Verification items for the finished model (mm, model axes). A direction names the side the tool comes from. Coordinates: 2 decimals unless noted, no trailing zeros. Order: outer loops, then holes, each group sorted by start corner. A loop starts at its lowest first (then second) coordinate and runs counter-clockwise, first axis right, second up. Notation, with made-up numbers: (55, -3) - (68, -3) arc R28 ccw to (68, 36) - close; hole circle Ø1 at (24, 67). An arc over 180 degrees is marked (long way). Answer as CSV lines item,"result". Start each with the question number.
1. Material ranges on L1, parallel to Y at x = 21.05, z = -28.5; L2, parallel to X at y = 9, z = -33; L3, parallel to Z at x = -3.5, y = 6.75, recorded low to high. Write a range as [from, to].
2. Section check C-C (z = -28.5). Record the cut outline in (x, y), and give its area (3 significant figures).
3. Section check A-A (z = -15.5). Record the cut outline in (x, y).
4. Section check B-B (y = 12.5). Record the cut outline in (x, z).
5. Set-up check for faces 4 (the cylindrical face through (20.857, 18.835, -32.206)), 5 (the cylindrical face through (-20.9, 12.68, -1.07)): record each of +Z, -Z, +X, -X, +Y, -Y from which the full face is reachable in a straight line by a thin tool's end or side.
6. Go/stop test with a flat-tipped pin: pin 1 (1.5 mm diameter, centred on x = -5, y = 21.5, fed in from -Z). Record where the tip stops, or that it passes through.
7. Mould release check, pull along Y, two halves, no side actions. Record for faces 1 (the cylindrical face through (-21.993, 18.835, -32.206)), 2 (the flat face through (21.35, 12, -21)), 3 (the flat face through (0, 0, 0)): pulls with the +Y half, pulls with the -Y half, needs draft (parallel to the pull), parting line crosses it, or undercut.
8. Section check D-D (z = -38). Count the separate pieces of the cut face and the enclosed holes in it, and give its area (3 significant figures).
from build123d import *

# Parameters (mm, degrees)
BOSS_EXTRUDE1_DEPTH = 25
SKETCH2_R           = 1
SKETCH2_R_2         = 6
CUT_EXTRUDE1_DEPTH  = 44.85
FILLET2_R           = 2
SKETCH3_R           = 1
CUT_EXTRUDE2_DEPTH  = 42


with BuildPart() as part:
    # Sketch1 → Boss-Extrude1 (new body)
    with BuildSketch(Plane(origin=(0, 0, 0), x_dir=(1, 0, 0), z_dir=(0, 1, 0))):
        Polygon((-21.5, 0.5), (20.35, 0.5), (20.35, 40.5), (21.35, 40.5), (21.35, 0.5), (21.35, -0.5), (-22.5, -0.5), (-22.5, 0.5), (-22.5, 40.5), (-21.5, 40.5), align=None)
    extrude(amount=BOSS_EXTRUDE1_DEPTH)

    # Sketch2 → Cut-Extrude1 (cut, through all)
    with BuildSketch(Plane(origin=(21.35, 0, 0), x_dir=(0, 0, -1), z_dir=(1, 0, 0))):
        with Locations((28.5, 12.5)):
            Circle(SKETCH2_R)
        with Locations((38, 12.5)):
            Circle(SKETCH2_R_2)
        with Locations((31.282485579, 19.217514421)):
            Circle(SKETCH2_R)
        with Locations((38, 22)):
            Circle(SKETCH2_R)
        with Locations((38, 3)):
            Circle(SKETCH2_R)
        with Locations((31.282485579, 5.782485579)):
            Circle(SKETCH2_R)
    extrude(amount=-CUT_EXTRUDE1_DEPTH, mode=Mode.SUBTRACT)

    # Fillet2
    fillet2_edges = [part.edges().sort_by_distance(p)[0] for p in [
        (21.35, 12.5, 0.5),
        (-22.5, 12.5, 0.5),
        (-21.5, 12.5, -0.5),
        (20.35, 12.5, -0.5),
    ]]
    fillet(fillet2_edges, radius=FILLET2_R)

    # Sketch3 → Cut-Extrude2 (cut, through all)
    with BuildSketch(Plane.XY.offset(0.5)):
        with Locations((-10.075, 20.585)):
            Circle(SKETCH3_R)
        with Locations((8.925, 20.585)):
            Circle(SKETCH3_R)
        with Locations((-10.075, 4.415)):
            Circle(SKETCH3_R)
        with Locations((8.925, 4.415)):
            Circle(SKETCH3_R)
    extrude(amount=-CUT_EXTRUDE2_DEPTH, mode=Mode.SUBTRACT)


solid = part.part
Evaluation:
1,L1,"y = [0, 11.5], [13.5, 25]"
1,L2,"x = [-22.5, -21.5], [20.35, 21.35]"
1,L3,"z = [-0.5, 0.5]"
2,outline,"(-22.5, 0) - (-21.5, 0) - (-21.5, 11.5) - (-22.5, 11.5) - close; (-22.5, 13.5) - (-21.5, 13.5) - (-21.5, 25) - (-22.5, 25) - close; (20.35, 0) - (21.35, 0) - (21.35, 11.5) - (20.35, 11.5) - close; (20.35, 13.5) - (21.35, 13.5) - (21.35, 25) - (20.35, 25) - close"
2,area,"46.0 mm²"
3,outline,"(-22.5, 0) - (-21.5, 0) - (-21.5, 25) - (-22.5, 25) - close; (20.35, 0) - (21.35, 0) - (21.35, 25) - (20.35, 25) - close"
4,outline,"(-22.5, -32) - (-21.5, -32) - (-21.5, -29.5) - (-22.5, -29.5) - close; (-22.5, -27.5) - (-21.5, -27.5) - (-21.5, -2.5) arc R2 cw to (-19.5, -0.5) - (18.35, -0.5) arc R2 cw to (20.35, -2.5) - (20.35, -27.5) - (21.35, -27.5) - (21.35, -1.5) arc R2 ccw to (19.35, 0.5) - (-20.5, 0.5) arc R2 ccw to (-22.5, -1.5) - close; (20.35, -32) - (21.35, -32) - (21.35, -29.5) - (20.35, -29.5) - close"
5,face 4,"+X, -X"
5,face 5,"-Z, +Y, -Y"
6,pin 1,"stops at z = -0.5"
7,face 1,"undercut"
7,face 2,"needs draft"
7,face 3,"pulls with the -Y half"
8,separate pieces,"8"
8,enclosed holes,"0"
8,area,"18.0 mm²"
